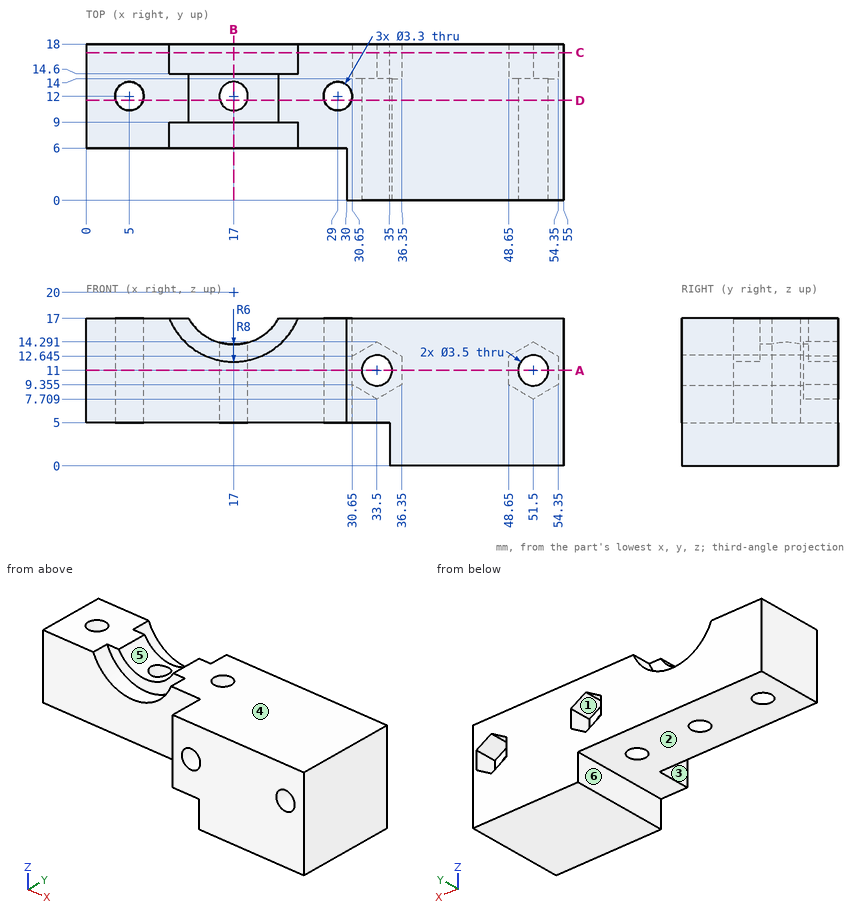
Study the drawing (mm; zero at the part's minimum x, y, z) and answer. A direction names the side the tool comes from. Coordinates: 2 decimals unless noted, no trailing zeros. Write each loop counter-clockwise with the first axis right and the second up, starting at its lowest first coordinate (ties: lowest second). Pieces come first, ordered by that corner, then holes. Notation, with made-up numbers: (16.25, -4) - (58.25, -4) arc R22 cw to (58.25, 26) - close; hole circle Ø5 at (46.25, 5.5). An arc over 180 degrees is marked (long way). Answer as a JSON object with one key per item and string values. Group by question number.
1. Consider L1, parallel to X at y = 9, z = 10.75; L2, parallel to X at y = 11.25, z = 15.25 (1 decimal); L3, parallel to Z at x = 33.5, y = 9.25. Determine where each line is inside the solid, lowest interval first. Write a range as [from, to].
2. A cutting plane is placed at D-D (y = 11.5). Determine the outline of the cut face in (x, z).
3. A cutting plane is placed at C-C (y = 17). Give the number of separate pieces and of enclosed holes in the cut face, plus the area to 3 significant figures.
4. Each of these flat-tipped pins is pushed along its axis until it touches: P1, Ø4, axis at y = 3.5, z = 15, coming from the -X side; P2, Ø5.5, axis at x = 51.5, z = 11, coming from the +Y side; P3, Ø5.5, axis at y = 13.5, z = 2, coming from the -X side; P4, Ø2, axis at x = 29, y = 12, coming from the -Z side. Where does it stop, or does it pass through?
5. A cutting plane is placed at B-B (x = 17). Determine the outline of the cut face in (y, z), plus the area to 3 significant figures.
6. The mould has two halves that part along X. Classify the marked faces 4, 5 and 6: +X half, -X half, draft (parallel to the pull), parting line (faces both ways), or undercut.
7. A cutting plane is placed at A-A (z = 11). Determine the outline of the cut face in (x, y), plus the area to 3 significant figures.
8. Which of the six approach directions +Z, -Z, +X, -X, +Y, -Y give full straight-line access (tool end or side, diameter ignored) to the marked faces 1, 2 and 3?
Worked out:
{
 "1": {"L1": "x = [0, 31.77], [35.23, 49.77], [53.23, 55]", "L2": "x = [0, 3.5], [6.5, 13.3], [20.7, 27.5], [30.5, 55]", "L3": "z = [5, 9.25], [12.75, 17]"},
 "2": {"outline": "(0, 5) - (3.43, 5) - (3.43, 17) - (0, 17) - close; (6.57, 5) - (15.43, 5) - (15.43, 14.21) arc R6 cw to (11.8, 17) - (6.57, 17) - close; (18.57, 5) - (27.43, 5) - (27.43, 17) - (22.2, 17) arc R6 cw to (18.57, 14.21) - close; (30.57, 5) - (35, 5) - (35, 0) - (55, 0) - (55, 17) - (30.57, 17) - close; hole circle Ø3.5 at (33.5, 11); hole circle Ø3.5 at (51.5, 11)"},
 "3": {"separate pieces": "1", "enclosed holes": "2", "area": "650 mm²"},
 "4": {"P1": "stops at x = 30", "P2": "stops at y = 14", "P3": "stops at x = 35", "P4": "passes through"},
 "5": {"outline": "(6, 5) - (10.35, 5) - (10.35, 14) - (9, 14) - (9, 12) - (6, 12) - close; (13.65, 5) - (18, 5) - (18, 12) - (14.6, 12) - (14.6, 14) - (13.65, 14) - close", "area": "65.5 mm²"},
 "6": {"face 4": "draft", "face 5": "undercut", "face 6": "-X half"},
 "7": {"outline": "(0, 6) - (30, 6) - (30, 0) - (31.75, 0) - (31.75, 14) - (30.65, 14) - (30.65, 18) - (0, 18) - close; (35.25, 0) - (49.75, 0) - (49.75, 14) - (48.65, 14) - (48.65, 18) - (36.35, 18) - (36.35, 14) - (35.25, 14) - close; (53.25, 0) - (55, 0) - (55, 18) - (54.35, 18) - (54.35, 14) - (53.25, 14) - close; hole circle Ø3.3 at (5, 12); hole circle Ø3.3 at (17, 12); hole circle Ø3.3 at (29, 12)", "area": "641 mm²"},
 "8": {"face 1": "+Y", "face 2": "-Z, -X, +Y, -Y", "face 3": "+Z, -Z, -X, -Y"}
}
